from build123d import *

# Parameters (mm, degrees)
SKETCH2_R                       = 65.405
BOSS_EXTRUDE1_DEPTH             = 6.35
SKETCH4_R                       = 65.405
SKETCH4_R_2                     = 61.976
CUT_EXTRUDE1_DEPTH              = 3.175
F_1_4_0_25_DIAMETER_HOLE1_D     = 6.35
F_13_16_0_8125_DIAMETER_HOLE1_D = 20.6375
CUT_EXTRUDE3_DEPTH              = 3.175
SKETCH9_R                       = 6.0325
CUT_EXTRUDE2_DEPTH              = 1.5875


with BuildPart() as part:
    # Sketch2 → Boss-Extrude1 (new body)
    with BuildSketch(Plane(origin=(0, 0, 0), x_dir=(1, 0, 0), z_dir=(0, 1, 0))):
        Circle(SKETCH2_R)
    extrude(amount=BOSS_EXTRUDE1_DEPTH)

    # Sketch4 → Cut-Extrude1 (cut)
    with BuildSketch(Plane(origin=(0, 6.35, 0), x_dir=(1, 0, 0), z_dir=(0, 1, 0))):
        Circle(SKETCH4_R)
        Circle(SKETCH4_R_2, mode=Mode.SUBTRACT)
    extrude(amount=-CUT_EXTRUDE1_DEPTH, mode=Mode.SUBTRACT)

    # 1/4 (0.25) Diameter Hole1 (through all)
    with Locations(Plane(origin=(0, 6.35, 0), x_dir=(1, 0, 0), z_dir=(0, 1, 0))):
        with Locations((-33.675960454, 33.675960454), (-33.675960454, -33.675960454), (33.675960454, 33.675960454), (33.675960454, -33.675960454)):
            Hole(F_1_4_0_25_DIAMETER_HOLE1_D / 2)

    # 13/16 (0.8125) Diameter Hole1 (through all)
    with Locations(Plane(origin=(0, 6.35, 0), x_dir=(1, 0, 0), z_dir=(0, 1, 0))):
        with Locations((0, 0)):
            Hole(F_13_16_0_8125_DIAMETER_HOLE1_D / 2)

    # Sketch11 → Cut-Extrude3 (cut)
    with BuildSketch(Plane(origin=(0, 6.35, 0), x_dir=(1, 0, 0), z_dir=(0, 1, 0))):
        with BuildLine():
            Line((-5.601020514, 10.2), (5.601020514, 10.2))
            ThreePointArc((5.601020514, 10.2), (7.490842879, 10.570899501), (9.100291576, 11.628571429))
            ThreePointArc((9.100291576, 11.628571429), (11.914213562, 11.614213562), (11.928571429, 8.800291576))
            ThreePointArc((11.928571429, 8.800291576), (10.870899501, 7.190842879), (10.5, 5.301020514))
            Line((10.5, 5.301020514), (10.5, -25.901020514))
            ThreePointArc((10.5, -25.901020514), (10.870899501, -27.790842879), (11.928571429, -29.400291576))
            ThreePointArc((11.928571429, -29.400291576), (11.914213562, -32.214213562), (9.100291576, -32.228571429))
            ThreePointArc((9.100291576, -32.228571429), (7.490842879, -31.170899501), (5.601020514, -30.8))
            Line((5.601020514, -30.8), (-5.601020514, -30.8))
            ThreePointArc((-5.601020514, -30.8), (-7.490842879, -31.170899501), (-9.100291576, -32.228571429))
            ThreePointArc((-9.100291576, -32.228571429), (-11.914213562, -32.214213562), (-11.928571429, -29.400291576))
            ThreePointArc((-11.928571429, -29.400291576), (-10.870899501, -27.790842879), (-10.5, -25.901020514))
            Line((-10.5, -25.901020514), (-10.5, 5.301020514))
            ThreePointArc((-10.5, 5.301020514), (-10.870899501, 7.190842879), (-11.928571429, 8.800291576))
            ThreePointArc((-11.928571429, 8.800291576), (-11.914213562, 11.614213562), (-9.100291576, 11.628571429))
            ThreePointArc((-9.100291576, 11.628571429), (-7.490842879, 10.570899501), (-5.601020514, 10.2))
        make_face()
    extrude(amount=-CUT_EXTRUDE3_DEPTH, mode=Mode.SUBTRACT)

    # Sketch9 → Cut-Extrude2 (cut)
    with BuildSketch(Plane.XZ):
        with Locations((-33.675960454, 33.675960454)):
            Circle(SKETCH9_R)
        with Locations((33.675960454, 33.675960454)):
            Circle(SKETCH9_R)
        with Locations((33.675960454, -33.675960454)):
            Circle(SKETCH9_R)
        with Locations((-33.675960454, -33.675960454)):
            Circle(SKETCH9_R)
    extrude(amount=-CUT_EXTRUDE2_DEPTH, mode=Mode.SUBTRACT)


solid = part.part
Could you check a few things on this model? Use its own coordinates, in mm. A direction names the side the tool comes from. Give positions to 0.01 mm unless a question says otherwise; leave off trailing zeros. Write each loop counter-clockwise with the first axis right and the second up, starting at its lowest first coordinate (ties: lowest second). Pieces come first, ordered by that corner, then holes. Notation, with made-up numbers: (-4, -19.75) -> (41, -19.75) arc R25 cw to (41, 12.25) -> close; hole circle Ø2 at (-25.75, 76). An arc over 180 degrees is marked (long way). Write each question's results on one line, items separated by ' | '. Start each with the question number.
Q1. Suppose I cut it at D-D, the plane z = 19. List the corners of the cut face in (x, y) for me (3 decimals), and give its area (3 significant figures).
Q2. We'd pull the mould along X, two halves only. Please class faces 1 (the face through (32.368, 0.783, 27.787)), 2 (the face through (-14.18, 1.57, 63.85)): +X half, -X half, draft (parallel to the pull), parting line (faces both ways), or undercut.
Q3. Suppose I cut it at B-B, the plane x = -46.5. List the corners of the cut face in (y, z) for me (3 decimals).
Q4. Suppose I cut it at A-A, the plane z = 0. List the corners of the cut face in (x, y) for me (3 decimals).
Q5. Suppose I cut it at C-C, the plane z = 45. List the corners of the cut face in (x, y) for me (3 decimals).
Q6. I need wall thicknesses on probe 1 along Z at (x, y) = (0, 2.75) (3 decimals); probe 2 along X at (y, z) = (3.75, -1); probe 3 along X at (y, z) = (1.5, -33.5). Which ranges of each line are inside material? Lowest first, please.
Q7. I'm going to push flat-ended pins straight in: pin 1 Ø6 at (x, z) = (35.5, 34.5) entering from -Y; pin 2 Ø2 at (y, z) = (2.5, -39.5) entering from +X; pin 3 Ø1 at (x, y) = (-22.5, 3.5) entering from +Z. Where does each tip first touch, or does it pass through?
Q8. Which directions (+Z, -Z, +X, -X, +Y, -Y) give clear straight access to the entire face, cutting with the end or side of a thin tool? Please do faces 3 (the face through (-35.383, 3.935, -36.353)), 4 (the face through (-31, 1.588, -36)), 5 (the face through (-10.881, 4.785, 27.816)).
Outcome:
1) outline: (-62.584, 0) -> (62.584, 0) -> (62.584, 3.175) -> (58.992, 3.175) -> (58.992, 6.35) -> (10.5, 6.35) -> (10.5, 3.175) -> (-10.5, 3.175) -> (-10.5, 6.35) -> (-58.992, 6.35) -> (-58.992, 3.175) -> (-62.584, 3.175) -> close | area: 705 mm2
2) face 1: undercut | face 2: parting line
3) outline: (0, -45.995) -> (3.175, -45.995) -> (3.175, -40.973) -> (6.35, -40.973) -> (6.35, 40.973) -> (3.175, 40.973) -> (3.175, 45.995) -> (0, 45.995) -> close
4) outline: (-65.405, 0) -> (-10.319, 0) -> (-10.319, 3.175) -> (-10.5, 3.175) -> (-10.5, 6.35) -> (-61.976, 6.35) -> (-61.976, 3.175) -> (-65.405, 3.175) -> close; (10.319, 0) -> (65.405, 0) -> (65.405, 3.175) -> (61.976, 3.175) -> (61.976, 6.35) -> (10.5, 6.35) -> (10.5, 3.175) -> (10.319, 3.175) -> close
5) outline: (-47.464, 0) -> (47.464, 0) -> (47.464, 3.175) -> (42.615, 3.175) -> (42.615, 6.35) -> (-42.615, 6.35) -> (-42.615, 3.175) -> (-47.464, 3.175) -> close
6) probe 1: -65.405 to -10.319, 10.319 to 65.405 | probe 2: -61.97 to -10.5, 10.5 to 61.97 | probe 3: -56.17 to -39.71, -27.65 to 27.65, 39.71 to 56.17
7) pin 1: y = 1.59 | pin 2: x = 52.87 | pin 3: z = 61.55
8) face 3: +Y, -Y | face 4: -Y | face 5: +Y
